from build123d import *

# Parameters (mm, degrees)
SKETCH1_R              = 17.5
SKETCH1_R_2            = 1.989574321
BOSS_EXTRUDE1_DEPTH    = 2
EXTRUDE_THIN1_START    = -9.5
SKETCH1_3_R            = 17.5
SKETCH1_3_R_2          = 15.5
EXTRUDE_THIN1_DEPTH    = 11.5
BOSS_EXTRUDE2_START    = -9.5
SKETCH1_4_W            = 0.2
SKETCH1_4_H            = 2.8
BOSS_EXTRUDE2_DEPTH    = 9.5
CUT_EXTRUDE1_START     = -11.064631417
CUT_EXTRUDE1_OUTLINE_W = 22
CUT_EXTRUDE1_OUTLINE_H = 5.5
CUT_EXTRUDE1_DEPTH     = 11.064631417


# Read off the part's stored shape, not the designer's step: Cut-Extrude1
with BuildPart() as part:
    # Sketch1 → Boss-Extrude1 (new body)
    with BuildSketch(Plane(origin=(0, 0, 0), x_dir=(1, 0, 0), z_dir=(0, 1, 0))):
        Polygon((-18.1, -16.016775893), (-12.131979642, -21.984796251), (11.942572252, -21.984796251), (18.1, -16.016073287), (18.1, -1.4), (18.3, -1.4), (18.3, 1.4), (18.1, 1.4), (18.1, 16.016073287), (11.932319604, 21.984796251), (-11.943274858, 21.984796251), (-18.1, 16.01675436), (-18.1, 1.4), (-18.3, 1.4), (-18.3, -1.4), (-18.1, -1.4), align=None)
        with Locations(Location((0, 0, 0), (0, 0, 270))):
            Circle(SKETCH1_R, mode=Mode.SUBTRACT)
        with Locations(Location((-14.8230313, -15.717637138, 0), (0, 0, 270))):
            Circle(SKETCH1_R_2, mode=Mode.SUBTRACT)
        with Locations(Location((15.02058352, -15.717637138, 0), (0, 0, 270))):
            Circle(SKETCH1_R_2, mode=Mode.SUBTRACT)
        with Locations(Location((-14.8230313, 14.432362862, 0), (0, 0, 270))):
            Circle(SKETCH1_R_2, mode=Mode.SUBTRACT)
        with Locations(Location((15.02058352, 14.432362862, 0), (0, 0, 270))):
            Circle(SKETCH1_R_2, mode=Mode.SUBTRACT)
    extrude(amount=BOSS_EXTRUDE1_DEPTH)

    # Sketch1<3> → Extrude-Thin1 (add)
    with BuildSketch(Plane(origin=(0, 0, 0), x_dir=(1, 0, 0), z_dir=(0, 1, 0)).offset(EXTRUDE_THIN1_START)):
        Circle(SKETCH1_3_R)
        Circle(SKETCH1_3_R_2, mode=Mode.SUBTRACT)
    extrude(amount=EXTRUDE_THIN1_DEPTH)

    # Sketch1<4> → Boss-Extrude2 (add)
    with BuildSketch(Plane(origin=(0, 0, 0), x_dir=(1, 0, 0), z_dir=(0, 1, 0)).offset(BOSS_EXTRUDE2_START)):
        with Locations((-18.2, 0)):
            Rectangle(SKETCH1_4_W, SKETCH1_4_H)
        with Locations((18.2, 0)):
            Rectangle(SKETCH1_4_W, SKETCH1_4_H)
        with BuildLine():
            ThreePointArc((17.5, 0), (17.485971906, -0.700561574), (17.443910112, -1.4))
            Line((17.443910112, -1.4), (18.1, -1.4))
            Line((18.1, -1.4), (18.1, 1.4))
            Line((18.1, 1.4), (17.443910112, 1.4))
            ThreePointArc((17.443910112, 1.4), (17.485971906, 0.700561574), (17.5, 0))
        make_face()
        with BuildLine():
            Line((-18.1, 1.4), (-18.1, -1.4))
            Line((-18.1, -1.4), (-17.443910112, -1.4))
            ThreePointArc((-17.443910112, -1.4), (-17.5, 0), (-17.443910112, 1.4))
            Line((-17.443910112, 1.4), (-18.1, 1.4))
        make_face()
    extrude(amount=BOSS_EXTRUDE2_DEPTH)

    # Cut-Extrude1 outline → Cut-Extrude1 (cut)
    with BuildSketch(Plane.XY.offset(21.984796251).offset(CUT_EXTRUDE1_START)):
        with Locations((0, -0.75)):
            Rectangle(CUT_EXTRUDE1_OUTLINE_W, CUT_EXTRUDE1_OUTLINE_H)
    extrude(amount=CUT_EXTRUDE1_DEPTH, mode=Mode.SUBTRACT)


solid = part.part
Can you work these out from the model? Positions are in its coordinate system, mm. A direction names the side the tool comes from. Give positions to 0.01 mm unless a question says otherwise; leave off trailing zeros. Loops run counter-clockwise (first coordinate to the right, second up) from the corner with the lowest first, then second, coordinate; pieces in that order, holes last. Notation, with made-up numbers: (38.5, 38.25) -> (62.5, 38.25) arc R21 ccw to (62.5, 52.25) -> close; hole circle Ø2 at (30, -22.75). An arc over 180 degrees is marked (long way). Use one line per item in the form item = value.
1) If we section it at B-B (z = 0): Please give me the cut outline in (x, y).
Answers:
outline = (-18.3, -9.5) -> (-15.5, -9.5) -> (-15.5, 2) -> (-18.3, 2) -> close; (15.5, -9.5) -> (18.3, -9.5) -> (18.3, 2) -> (15.5, 2) -> close
2) If we section it at D-D (x = -14): Please give me the cut outline in (y, z), plus the area to 3 significant figures.
Answers:
outline = (-9.5, -10.5) -> (0, -10.5) -> (0, -12.62) -> (2, -12.62) -> (2, -6.65) -> (-9.5, -6.65) -> close; (-9.5, 6.65) -> (2, 6.65) -> (2, 13.91) -> (0, 13.91) -> (0, 10.5) -> (-9.5, 10.5) -> close; (0, -19.99) -> (2, -19.99) -> (2, -16.24) -> (0, -16.24) -> close; (0, 17.53) -> (2, 17.53) -> (2, 20.12) -> (0, 20.12) -> close
area = 112 mm²
3) I need wall thicknesses on line 1 along X through (y, z) = (-2.75, 0); line 2 along Z through (x, y) = (0, -4.75); line 3 along Y through (x, z) = (-14.5, -12). Which ranges of each line are inside material? Lowest first, please.
Answers:
line_1 = -18.3 to -15.5, 15.5 to 18.3
line_2 = -17.5 to -15.5, 15.5 to 17.5
line_3 = 0 to 2
4) If we section it at A-A (x = 0): Please give me the cut outline in (y, z).
Answers:
outline = (-9.5, -17.5) -> (0, -17.5) -> (0, -21.98) -> (2, -21.98) -> (2, -15.5) -> (-9.5, -15.5) -> close; (-9.5, 15.5) -> (-3.5, 15.5) -> (-3.5, 17.5) -> (-9.5, 17.5) -> close
5) For faces 1 (the face through (0.365, -4.816, -17.496)), 2 (the face through (-0.365, -5.872, 17.496)), 3 (the face through (11, 0.4, 15.1)), which set-ups out of +Z, -Z, +X, -X, +Y, -Y let a thin tool reach every point of the face, with its end or its side?
Answers:
face_1 = -Z, -Y
face_2 = +Z, -Y
face_3 = +Z, +Y
6) Will these pins go through, and if not, where does the flat tip stop? pin 1 (5.5 mm diameter, centred on x = 13.5, z = 16.5, fed in from -Y); pin 2 (1.6 mm diameter, centred on y = 0.5, z = 14.5, fed in from +X); pin 3 (0.7 mm diameter, centred on x = -18, y = -3.5, fed in from +Z); pin 4 (3 mm diameter, centred on x = 15.02, z = 15.72, fed in from +Y).
Answers:
pin_1 = 0
pin_2 = 18.1
pin_3 = 1.4
pin_4 = through
